The listing builds one solid part. Answer for the finished solid, in the listing's coordinates (mm). Face numbers are marked on the shaded views. A direction names the side the tool comes from. Coordinates: 2 decimals unless noted, no trailing zeros. Order: outer loops, then holes, each group sorted by start corner. A loop starts at its lowest first (then second) coordinate and runs counter-clockwise, first axis right, second up.
from build123d import *

# Parameters (mm, degrees)
SKETCH1_W           = 19.05
SKETCH1_H           = 10.16
SKETCH1_R           = 2.2
SKETCH1_W_2         = 2.9972
SKETCH1_H_2         = 2.9972
BOSS_EXTRUDE1_DEPTH = 2.9972
FILLET1_R           = 3.175


with BuildPart() as part:
    # Sketch1 → Boss-Extrude1 (new body)
    with BuildSketch(Plane(origin=(0, 0, 0), x_dir=(1, 0, 0), z_dir=(0, 1, 0))):
        with Locations((9.525, 5.08)):
            Rectangle(SKETCH1_W, SKETCH1_H)
        with Locations(Location((5.08, 5.08, 0), (0, 0, 90))):
            Circle(SKETCH1_R, mode=Mode.SUBTRACT)
        with Locations((14.3764, 2.5654)):
            Rectangle(SKETCH1_W_2, SKETCH1_H_2, mode=Mode.SUBTRACT)
        with Locations((14.3764, 7.5946)):
            Rectangle(SKETCH1_W_2, SKETCH1_H_2, mode=Mode.SUBTRACT)
    extrude(amount=BOSS_EXTRUDE1_DEPTH)

    # Fillet1
    fillet1_edges = [part.edges().sort_by_distance(p)[0] for p in [
        (0, 1.4986, -10.16),
        (19.05, 1.4986, -10.16),
        (19.05, 1.4986, 0),
        (0, 1.4986, 0),
    ]]
    fillet(fillet1_edges, radius=FILLET1_R)


solid = part.part
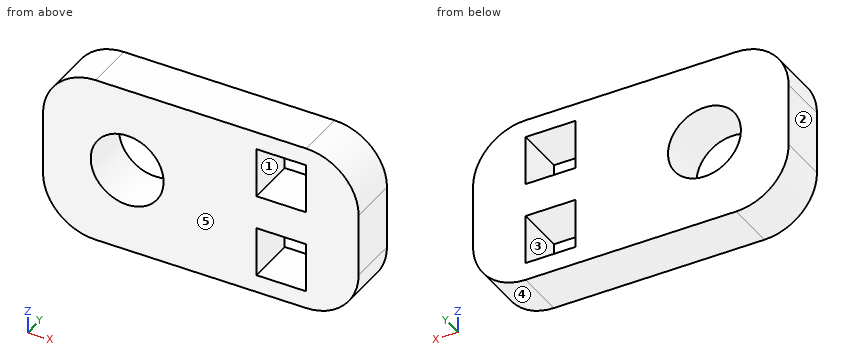
(1) Find the intervals of material crossed by probe 1 along Z at (x, y) = (14.5, 2.9); probe 2 along X at (y, z) = (0.9, -5.08); probe 3 along X at (y, z) = (1.75, -4) (3 decimals), in increasing order.
(2) Given pin 1 Ø1 at (y, z) = (2, -2) entering from -X, flat-ended and moving along its own axis, determine where the tip first touches the part or whether it passes through.
(3) Find section A-A on y = 2.2. Determine the outline of the cut face in (x, z) (3 decimals), then the cut area to 3 significant figures.
(4) A tool of negligible diameter and unlimited length cuts with its end or side. For the marked faces 1 and 2, from which of +Z, -Z, +X, -X, +Y, -Y can it reach the whole face along a straight path? Write none if from no direction.
(5) Find section C-C on x = 5.08. Determine the outline of the cut face in (y, z).
(6) The mould has two halves that part along Z. Classify the marked faces 3, 4 and 5: pulls with the +Z half, pulls with the -Z half, needs draft (parallel to the pull), parting line crosses it, or undercut.
(7) Find section D-D on x = 17.5. Determine the outline of the cut face in (y, z), then the cut area to 3 significant figures.
(8) Find section B-B on z = -5.08. Determine the outline of the cut face in (x, y).
Resolved:
1. probe 1: z = -10.16 to -9.09, -6.1 to -4.06, -1.07 to 0
1. probe 2: x = 0 to 2.88, 7.28 to 19.05
1. probe 3: x = 0 to 3.163, 6.997 to 12.878, 15.875 to 19.05
2. pin 1: stops at x = 0.07
3. outline: (0, -6.985) arc R3.175 ccw to (3.175, -10.16) - (15.875, -10.16) arc R3.175 ccw to (19.05, -6.985) - (19.05, -3.175) arc R3.175 ccw to (15.875, 0) - (3.175, 0) arc R3.175 ccw to (0, -3.175) - close; hole circle Ø4.4 at (5.08, -5.08); hole (12.878, -9.093) - (15.875, -9.093) - (15.875, -6.096) - (12.878, -6.096) - close; hole (12.878, -4.064) - (15.875, -4.064) - (15.875, -1.067) - (12.878, -1.067) - close
3. area: 152 mm2
4. face 1: +Y, -Y
4. face 2: +Z, -Z, -X, +Y, -Y
5. outline: (0, -10.16) - (3, -10.16) - (3, -7.28) - (0, -7.28) - close; (0, -2.88) - (3, -2.88) - (3, 0) - (0, 0) - close
6. face 3: undercut
6. face 4: pulls with the -Z half
6. face 5: needs draft
7. outline: (0, -9.71) - (3, -9.71) - (3, -0.45) - (0, -0.45) - close
7. area: 27.8 mm2
8. outline: (0, 0) - (2.88, 0) - (2.88, 3) - (0, 3) - close; (7.28, 0) - (19.05, 0) - (19.05, 3) - (7.28, 3) - close
